Here's how the part is built. I have some questions about the finished solid (model axes, mm). Face numbers are marked on the shaded views. A direction names the side the tool comes from. Round coordinates to 2 decimals unless told otherwise and drop trailing zeros. Order: outer loops, then holes, each group sorted by start corner. A loop starts at its lowest first (then second) coordinate and runs counter-clockwise, first axis right, second up.
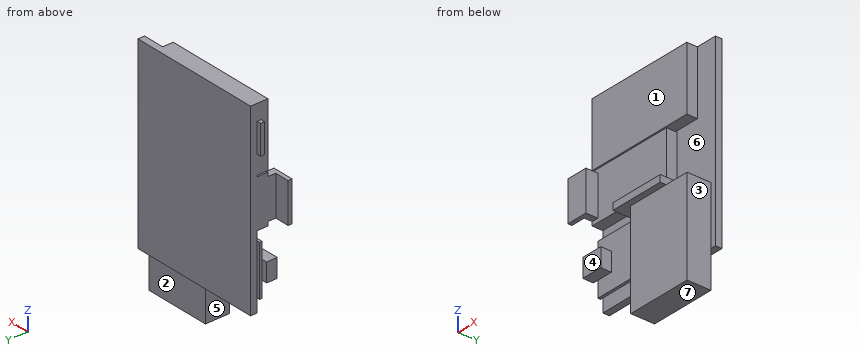
```python
from build123d import *

# Parameters (mm, degrees)
F0_W      = 50
F0_H      = 70
F1_DEPTH  = 1
F2_W      = 42
F2_H      = 24
F3_DEPTH  = 4
F4_W      = 25
F4_H      = 36
F5_DEPTH  = 9
F6_W      = 24
F6_H      = 19
F7_DEPTH  = 1
F8_W      = 8
F8_H      = 7
F9_DEPTH  = 4
F10_W     = 33
F10_H     = 18
F11_DEPTH = 4
F12_W     = 2.54
F12_H     = 15
F13_DEPTH = 3
F15_DEPTH = 15
F16_W     = 21
F16_H     = 2.54
F17_DEPTH = 8.5
F18_W     = 1.5
F18_H     = 11
F19_DEPTH = 1.5
F20_DEPTH = 1.5


with BuildPart() as f1:
    # F0 (on Front) → F1 (new body)
    with BuildSketch(Plane.XZ):
        Rectangle(F0_W, F0_H)
    extrude(amount=F1_DEPTH)

    # F2 (on face) → F3 (join)
    with BuildSketch(Plane.XZ.offset(1)):
        with Locations((-4, 23)):
            Rectangle(F2_W, F2_H)
    extrude(amount=F3_DEPTH)

    # F4 (on face) → F5 (join)
    with BuildSketch(Plane.XZ.offset(1)):
        with Locations((10.5, -31)):
            Rectangle(F4_W, F4_H)
    extrude(amount=F5_DEPTH)

    # F6 (on face) → F7 (join)
    with BuildSketch(Plane.XZ.offset(1)):
        with Locations((-14, -20.5)):
            Rectangle(F6_W, F6_H)
    extrude(amount=F7_DEPTH)

    # F8 (on face) → F9 (join)
    with BuildSketch(Plane.XZ.offset(2)):
        with Locations((-24, -20.5)):
            Rectangle(F8_W, F8_H)
    extrude(amount=F9_DEPTH)

    # F10 (on face) → F11 (join)
    with BuildSketch(Plane.XZ.offset(1)):
        with Locations((-8.5, 1.5)):
            Rectangle(F10_W, F10_H)
    extrude(amount=F11_DEPTH)

    # F12 (on face) → F13 (join)
    with BuildSketch(Plane.XZ.offset(5)):
        with Locations((-23.73, 1.5)):
            Rectangle(F12_W, F12_H)
    extrude(amount=F13_DEPTH)

    # F14 (on face) → F15 (join, through all)
    with BuildSketch(Plane(origin=(0, 0, -6), x_dir=(1, 0, 0), z_dir=(0, 0, -1))):
        Polygon((-22.46, 9.5), (-30.46, 9.5), (-30.46, 8), (-25, 8), (-22.46, 8), align=None)
    extrude(amount=-F15_DEPTH)

    # F16 (on face) → F17 (join)
    with BuildSketch(Plane.XZ.offset(1)):
        with Locations((0, -9.23)):
            Rectangle(F16_W, F16_H)
    extrude(amount=F17_DEPTH)

    # F18 (on face) → F19 (join)
    with BuildSketch(Plane(origin=(-25, 0, 0), x_dir=(0, -1, 0), z_dir=(-1, 0, 0))):
        with Locations((1.75, 23.5)):
            Rectangle(F18_W, F18_H)
    extrude(amount=F19_DEPTH)

    # F20 (add): a face of the model
    f20_faces = [f1.faces().sort_by_distance(p)[0] for p in [
        (0, 0, 0),
    ]]
    extrude(f20_faces, amount=F20_DEPTH)


solid = f1.part
```
1) I need wall thicknesses on line 1 (Z direction, x = 0, y = -4.75); line 2 (Z direction, x = -4, y = -1.25); line 3 (Z direction, x = 14, y = -1.5). Which ranges of each line are inside material? Lowest first, please.
2) We'd pull the mould along Z, two halves only. Please class the marked faces 5, 6 and 7: +Z half, -Z half, draft (parallel to the pull), parting line (faces both ways), or undercut.
3) For the marked faces 1, 2, 3 and 4, which set-ups out of +Z, -Z, +X, -X, +Y, -Y let a thin tool reach every point of the face, with its end or its side?
4) If we section it at A-A (y = -3.5): Write out the boundary of the cut face in (x, z), plus the area to 3 significant figures.
5) I'm going to push flat-ended pins straight in: pin 1 (2 mm diameter, centred on y = -2.5, z = 17.5, fed in from +X); pin 2 (1.5 mm diameter, centred on x = -2, z = -3.5, fed in from -Y); pin 3 (1.3 mm diameter, centred on y = -5, z = -9, fed in from -X). Where does each tip first touch, or does it pass through?
6) If we section it at C-C (x = 16): Write out the boundary of the cut face in (y, z), plus the area to 3 significant figures.
7) If we section it at B-B (z = -25): Write out the boundary of the cut face in (x, y).
8) If we section it at D-D (x = 0.5): Write out the boundary of the cut face in (y, z), plus the area to 3 significant figures.
Solutions:
1. line 1: z = -49 to -13, -10.5 to -7.96, -7.5 to 10.5, 11 to 35
1. line 2: z = -30 to -11, -10.5 to -7.96, -7.5 to 10.5, 11 to 35
1. line 3: z = -49 to -13, 11 to 35
2. face 5: draft
2. face 6: undercut
2. face 7: -Z half
3. face 1: +Z, +X, -X, -Y
3. face 2: -Z, +X, -X, +Y
3. face 3: +Z, -Z, +X, -Y
3. face 4: -Z, -X, -Y
4. outline: (-28, -24) - (-20, -24) - (-20, -17) - (-28, -17) - close; (-25, -7.5) - (8, -7.5) - (8, 10.5) - (-25, 10.5) - close; (-25, 11) - (17, 11) - (17, 35) - (-25, 35) - close; (-10.5, -10.5) - (10.5, -10.5) - (10.5, -7.96) - (-10.5, -7.96) - close; (-2, -49) - (23, -49) - (23, -13) - (-2, -13) - close
4. area: 2,610 mm2
5. pin 1: stops at x = 17
5. pin 2: stops at y = -5
5. pin 3: stops at x = -10.5
6. outline: (-10, -49) - (-1, -49) - (-1, -35) - (1.5, -35) - (1.5, 35) - (-5, 35) - (-5, 11) - (-1, 11) - (-1, -13) - (-10, -13) - close
6. area: 595 mm2
7. outline: (-26, -2) - (-2, -2) - (-2, -10) - (23, -10) - (23, -1) - (25, -1) - (25, 1.5) - (-25, 1.5) - (-25, -1) - (-26, -1) - close
8. outline: (-10, -49) - (-1, -49) - (-1, -35) - (1.5, -35) - (1.5, 35) - (-5, 35) - (-5, 11) - (-1, 11) - (-1, 10.5) - (-5, 10.5) - (-5, -7.5) - (-1, -7.5) - (-1, -7.96) - (-9.5, -7.96) - (-9.5, -10.5) - (-1, -10.5) - (-1, -13) - (-10, -13) - close
8. area: 689 mm2
